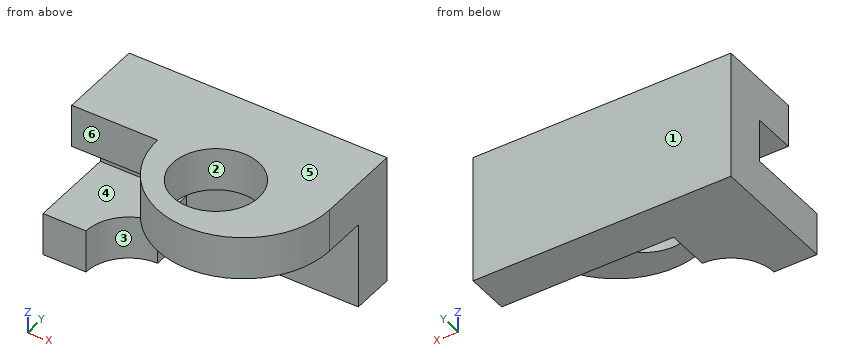
from build123d import *

# Parameters (mm, degrees)
F1_DEPTH  = 254
F0_W      = 508
F0_H      = 254
F2_DEPTH  = 762
F4_DEPTH  = 254
F5_W      = 1524
F5_H      = 254
F6_DEPTH  = 254
F8_DEPTH  = 254
F9_R      = 254
F10_DEPTH = 254


with BuildPart() as f1:
    # F0 (on Front) → F1 (new body)
    with BuildSketch(Plane.XZ):
        Polygon((0, 0), (0, -508), (508, -508), (508, -762), (1524, -762), (1524, 0), align=None)
    extrude(amount=F1_DEPTH)

    # F0 (on Front) → F2 (join)
    with BuildSketch(Plane.XZ):
        with Locations((254, -635)):
            Rectangle(F0_W, F0_H)
    extrude(amount=F2_DEPTH)

    # F3 (on face) → F4 (cut)
    with BuildSketch(Plane(origin=(0, 0, -762), x_dir=(1, 0, 0), z_dir=(0, 0, -1))):
        with BuildLine():
            ThreePointArc((254, 762), (328.394878, 582.394878), (508, 508))
            Line((508, 508), (508, 762))
            Line((508, 762), (254, 762))
        make_face()
    extrude(amount=-F4_DEPTH, mode=Mode.SUBTRACT)

    # F5 (on face) → F6 (join)
    with BuildSketch(Plane.XZ.offset(254)):
        with Locations((762, -127)):
            Rectangle(F5_W, F5_H)
    extrude(amount=F6_DEPTH)

    # F7 (on face) → F8 (join)
    with BuildSketch(Plane(origin=(0, 0, -254), x_dir=(1, 0, 0), z_dir=(0, 0, -1))):
        with BuildLine():
            Line((508, 508), (1524, 508))
            ThreePointArc((1524, 508), (1016, 1016), (508, 508))
        make_face()
    extrude(amount=-F8_DEPTH)

    # F9 (on face) → F10 (cut)
    with BuildSketch(Plane(origin=(0, 0, -254), x_dir=(1, 0, 0), z_dir=(0, 0, -1))):
        with Locations((925.507426, 617.637932)):
            Circle(F9_R)
    extrude(amount=-F10_DEPTH, mode=Mode.SUBTRACT)


solid = f1.part
Build history of the part. All positions in model axes, mm. Face numbers are marked on the shaded views. A direction names the side the tool comes from. Round coordinates to 2 decimals unless told otherwise and drop trailing zeros. Write each loop counter-clockwise with the first axis right and the second up, starting at its lowest first coordinate (ties: lowest second). Pieces come first, ordered by that corner, then holes. Notation, with made-up numbers: (47.25, 22) -> (65.25, 22) arc R26 ccw to (65.25, 46) -> close; hole circle Ø6 at (49.5, 46.25). An arc over 180 degrees is marked (long way). Write item = value, one per line.
(1) Band-saw the part on D-D (y = -559). Give the cut face in (x, z).
Answer:
outline = (0, -762) -> (355.33, -762) -> (355.33, -508) -> (0, -508) -> close; (510.57, -254) -> (678.37, -254) -> (678.37, 0) -> (510.57, 0) -> close; (1172.65, -254) -> (1521.43, -254) -> (1521.43, 0) -> (1172.65, 0) -> close
(2) Band-saw the part on C-C (z = -632). Give the cut face in (x, y).
Answer:
outline = (0, -762) -> (254, -762) arc R254 cw to (508, -508) -> (508, -254) -> (1524, -254) -> (1524, 0) -> (0, 0) -> close
(3) Probe L1, parallel to Z at x = 430, y = -491; L2, parallel to Y at x = 78.5, z = -682.5; L3, parallel to Y at x = 645, z = -463. List the from-to ranges inside material, lowest first.
Answer:
L1 = -762 to -508, -254 to 0
L2 = -762 to 0
L3 = -254 to 0
(4) Band-saw the part on A-A (y = -291). Give the cut face in (x, z).
Answer:
outline = (0, -762) -> (508, -762) -> (508, -508) -> (0, -508) -> close; (0, -254) -> (1524, -254) -> (1524, 0) -> (0, 0) -> close
(5) Two-plate mould, pull along X, no slides. Class the marked faces 1, 2 and 3: pulls with the +X half, pulls with the -X half, needs draft (parallel to the pull), parting line crosses it, or undercut.
Answer:
face_1 = needs draft
face_2 = undercut
face_3 = pulls with the +X half
(6) Tool access for the marked faces 4, 5 and 6: list every direction of +Z, -Z, +X, -X, +Y, -Y with a clear straight run to the whole face (end or side of a thin tool).
Answer:
face_4 = +X, -X, -Y
face_5 = +Z, +X, -X, +Y, -Y
face_6 = +Z, -X, -Y
(7) Flat gauge pins, fed straight in: pin 1 (2 mm diameter, centred on x = 1101, y = -876, fed in from -Z); pin 2 (4 mm diameter, centred on x = 602.5, z = -548.5, fed in from -Y); pin 3 (1.5 mm diameter, centred on y = -854.5, z = -232.5, fed in from +X). Where does each tip first touch, or does it go through?
Answer:
pin_1 = -254
pin_2 = -254
pin_3 = 1388.18
(8) Band-saw the part on B-B (x = 1054.5). Give the cut face in (y, z).
Answer:
outline = (-1014.54, -254) -> (-836.45, -254) -> (-836.45, 0) -> (-1014.54, 0) -> close; (-398.83, -254) -> (-254, -254) -> (-254, -762) -> (0, -762) -> (0, 0) -> (-398.83, 0) -> close
